```python
from build123d import *

# Parameters (mm, degrees)
SKETCH1_R           = 1.75
BOSS_EXTRUDE1_DEPTH = 10
SKETCH2_W           = 30
SKETCH2_H           = 30
BOSS_EXTRUDE2_DEPTH = 6
SKETCH3_W           = 2
SKETCH3_H           = 24.678853852
CUT_EXTRUDE1_DEPTH  = 28
BOSS_EXTRUDE3_DEPTH = 10
SKETCH5_W           = 6
SKETCH5_H           = 4
CUT_EXTRUDE2_DEPTH  = 6


with BuildPart() as part:
    # Sketch1 → Boss-Extrude1 (new body)
    with BuildSketch(Plane.XY):
        with BuildLine():
            ThreePointArc((-3, 0), (0, -3), (3, 0))
            Line((3, 0), (3, 70))
            Line((3, 70), (-3, 70))
            Line((-3, 70), (-3, 0))
        make_face()
        Circle(SKETCH1_R, mode=Mode.SUBTRACT)
    extrude(amount=BOSS_EXTRUDE1_DEPTH)

    # Sketch2 → Boss-Extrude2 (add)
    with BuildSketch(Plane.ZY.offset(3)):
        with Locations((5, 55)):
            Rectangle(SKETCH2_W, SKETCH2_H)
    extrude(amount=-BOSS_EXTRUDE2_DEPTH)

    # Sketch3 → Cut-Extrude1 (cut)
    with BuildSketch(Plane(origin=(0, 70, 0), x_dir=(1, 0, 0), z_dir=(0, 1, 0))):
        with Locations((-2, -5)):
            Rectangle(SKETCH3_W, SKETCH3_H)
        Polygon((-1, 8.839426926), (-1, 7.339426926), (-1, -17.339426926), (-1, -18.839426926), (0.5, -18.839426926), (0.5, 8.839426926), align=None)
    extrude(amount=-CUT_EXTRUDE1_DEPTH, mode=Mode.SUBTRACT)

    # Sketch4 → Boss-Extrude3 (add)
    with BuildSketch(Plane.XY.offset(10)):
        with BuildLine():
            ThreePointArc((9, 67), (8.121320344, 69.121320344), (6, 70))
            Line((6, 70), (6, 68.75))
            ThreePointArc((6, 68.75), (7.237436867, 68.237436867), (7.75, 67))
            ThreePointArc((7.75, 67), (7.237436867, 65.762563133), (6, 65.25))
            Line((6, 65.25), (6, 64))
            ThreePointArc((6, 64), (8.121320344, 64.878679656), (9, 67))
        make_face()
        with BuildLine():
            Line((6, 68.75), (6, 70))
            ThreePointArc((6, 70), (3.878679658, 69.121320346), (3, 67.000000006))
            ThreePointArc((3, 67.000000006), (3.878679654, 64.878679658), (6, 64))
            Line((6, 64), (6, 65.25))
            ThreePointArc((6, 65.25), (4.25, 67), (6, 68.75))
        make_face()
        with BuildLine():
            ThreePointArc((3, 67.000000006), (3.878679658, 69.121320346), (6, 70))
            Line((6, 70), (3, 70))
            Line((3, 70), (3, 67.000000006))
        make_face()
        with BuildLine():
            ThreePointArc((6, 64), (3.878679654, 64.878679658), (3, 67.000000006))
            Line((3, 67.000000006), (3, 64))
            Line((3, 64), (6, 64))
        make_face()
    extrude(amount=-BOSS_EXTRUDE3_DEPTH)

    # Sketch5 → Cut-Extrude2 (cut)
    with BuildSketch(Plane(origin=(0, 70, 0), x_dir=(1, 0, 0), z_dir=(0, 1, 0))):
        with Locations((6, -5)):
            Rectangle(SKETCH5_W, SKETCH5_H)
    extrude(amount=-CUT_EXTRUDE2_DEPTH, mode=Mode.SUBTRACT)


solid = part.part
```
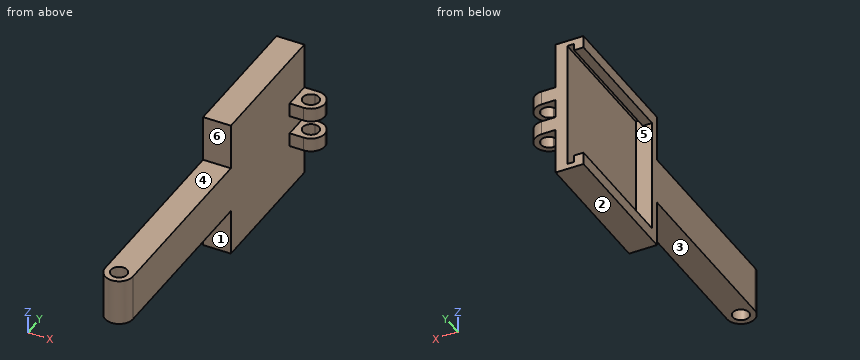
Here's how the part is built. I have some questions about the finished solid (model axes, mm). Face numbers are marked on the shaded views. A direction names the side the tool comes from. Coordinates: 2 decimals unless noted, no trailing zeros. Order: outer loops, then holes, each group sorted by start corner. A loop starts at its lowest first (then second) coordinate and runs counter-clockwise, first axis right, second up.
1) Imagine slicing it at C-C on z = -3.5. List the corners of the cut face in (x, y) for me.
2) Imagine slicing it at A-A on x = 6.75. List the corners of the cut face in (y, z) for me, and give its area (3 significant figures).
3) Which directions (+Z, -Z, +X, -X, +Y, -Y) give clear straight access to the entire face, cutting with the end or side of a thin tool? Please do the marked faces 1 and 2.
4) Imagine slicing it at D-D on y = 4. List the corners of the cut face in (x, z) for me, and give its area (3 significant figures).
5) We'd pull the mould along Z, two halves only. Please class the marked faces 3, 4, 5 and 6: +Z half, -Z half, draft (parallel to the pull), parting line (faces both ways), or undercut.
6) Will these pins go through, and if not, where does the flat tip stop? pin 1 (3 mm diameter, centred on x = 6.5, y = 66.5, fed in from +Z); pin 2 (1.6 mm diameter, centred on y = 50, z = 18, fed in from +X); pin 3 (8.5 mm diameter, centred on y = 62, z = 6.5, fed in from -X); pin 4 (2 mm diameter, centred on x = 5.5, z = 16.5, fed in from -Y).
7) Imagine slicing it at B-B on z = 4.75. List the corners of the cut face in (x, y) for me.
8) I need wall thicknesses on line 1 (Y direction, x = 0, z = 3.25); line 2 (X direction, y = 53.5, z = 17.5); line 3 (Z direction, x = -2, y = 65). Which ranges of each line are inside material? Lowest first, please.
Response values:
1. outline: (-3, 40) - (3, 40) - (3, 70) - (0.5, 70) - (0.5, 42) - (-3, 42) - close
2. outline: (64.1, 0) - (65.42, 0) - (65.42, 3) - (64.1, 3) - close; (64.1, 7) - (65.42, 7) - (65.42, 10) - (64.1, 10) - close; (68.58, 0) - (69.9, 0) - (69.9, 3) - (68.58, 3) - close; (68.58, 7) - (69.9, 7) - (69.9, 10) - (68.58, 10) - close
2. area: 15.9 mm2
3. face 1: -Z, +X, -X, -Y
3. face 2: -Z, +X, -X, +Y, -Y
4. outline: (-3, 0) - (3, 0) - (3, 10) - (-3, 10) - close
4. area: 60.0 mm2
5. face 3: -Z half
5. face 4: +Z half
5. face 5: undercut
5. face 6: draft
6. pin 1: stops at z = 10
6. pin 2: stops at x = 3
6. pin 3: stops at x = 0.5
6. pin 4: passes through
7. outline: (-3, 0) arc R3 ccw to (3, 0) - (3, 70) - (0.5, 70) - (0.5, 42) - (-3, 42) - close; hole circle Ø3.5 at (0, 0)
8. line 1: y = -3 to -1.75, 1.75 to 42
8. line 2: x = -3 to -1, 0.5 to 3
8. line 3: z = -10 to -7.34, 17.34 to 20
